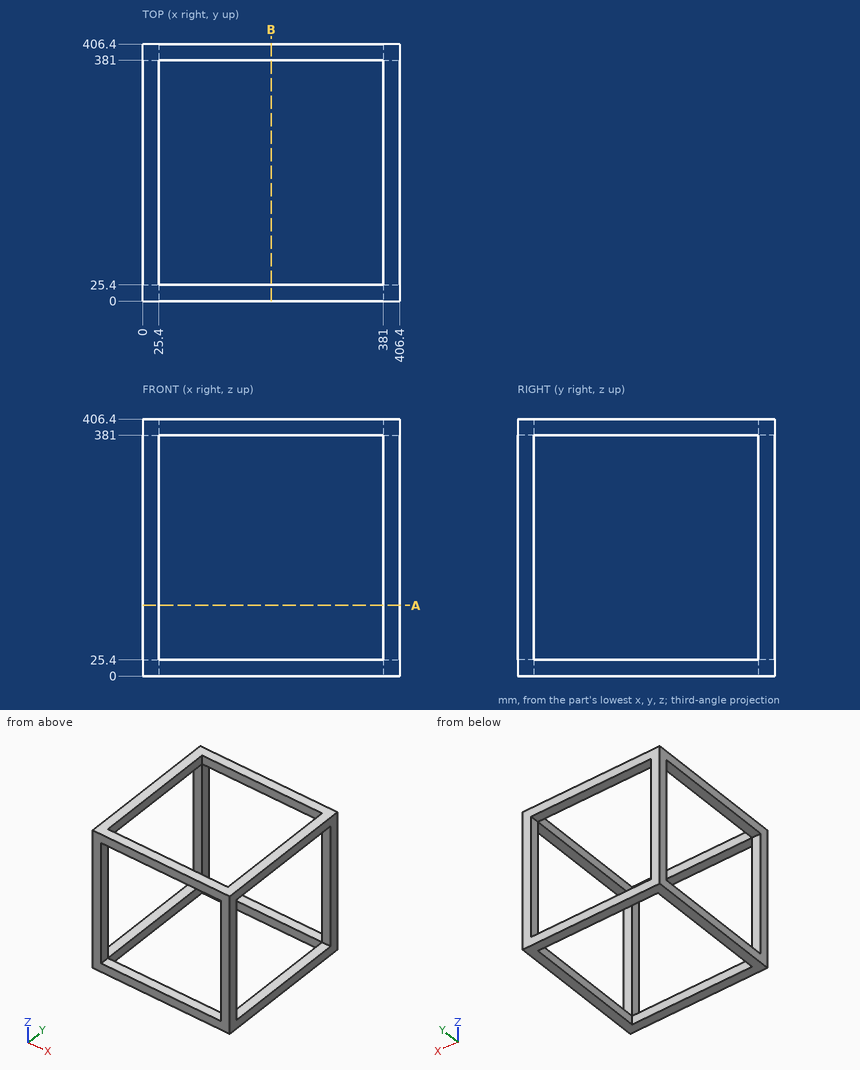
The figure shows three views and two pictorial views of one solid part (mm, origin at its lowest corner). Answer the questions. Coordinates: 2 decimals unless noted, no trailing zeros. Loops run counter-clockwise (first coordinate to the right, second up) from the corner with the lowest first, then second, coordinate; pieces in that order, holes last. Notation, with made-up numbers: (10.5, -34.5) -> (28.5, -34.5) arc R25 cw to (28.5, -8.5) -> close; hole circle Ø5 at (1.5, 73.25). An arc over 180 degrees is marked (long way). Write item = value, one per line. Start each with the question number.
1) A cutting plane is placed at A-A (z = 111.5). Give the vertices of the cut face in (x, y), then the cut area to 3 significant figures.
2) A straight line is drawn through the part: line 1 (Y direction, x = 21, z = 287). Find the intervals that lie inside material, in ascending order. Write a range as from..to.
Responses:
q1.outline = (0, 0) -> (25.4, 0) -> (25.4, 25.4) -> (0, 25.4) -> close; (0, 381) -> (25.4, 381) -> (25.4, 406.4) -> (0, 406.4) -> close; (381, 0) -> (406.4, 0) -> (406.4, 25.4) -> (381, 25.4) -> close; (381, 381) -> (406.4, 381) -> (406.4, 406.4) -> (381, 406.4) -> close
q1.area = 2,580 mm²
q2.line_1 = 0..25.4, 381..406.4
